Read the model definition and answer for the solid it produces. Units are mm, in the model's axes. Give positions to 0.01 mm unless a question says otherwise; leave off trailing zeros. Write each loop counter-clockwise with the first axis right and the second up, starting at its lowest first coordinate (ties: lowest second). Pieces come first, ordered by that corner, then holes. Notation, with made-up numbers: M -39,62.5 L -29,62.5 A20 cw -29,78.5 Z; hole C 74,51.5 d8. An arc over 180 degrees is marked long. Write each question's results on one line, items separated by ' | '. Start each with the question number.
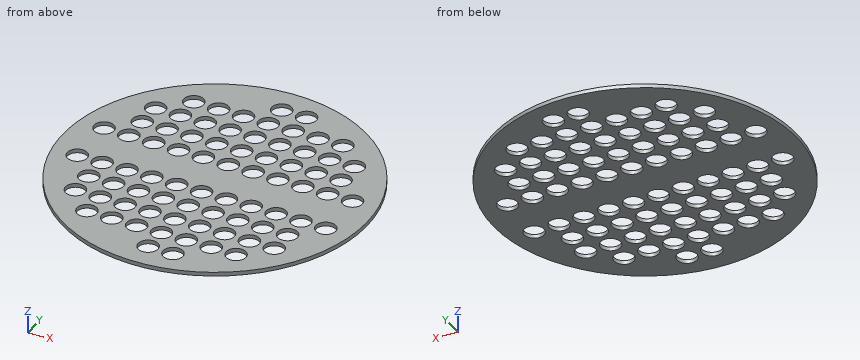
```python
from build123d import *

# Parameters (mm, degrees)
SKETCH1_R           = 193.65
BOSS_EXTRUDE1_DEPTH = 5
SKETCH2_R           = 12.7
CUT_EXTRUDE1_DEPTH  = 274.908095901


with BuildPart() as part:
    # Sketch1 → Boss-Extrude1 (new body)
    with BuildSketch(Plane.XY):
        Circle(SKETCH1_R)
    extrude(amount=BOSS_EXTRUDE1_DEPTH)

    # Sketch2 → Cut-Extrude1 (cut, through all)
    with BuildSketch(Plane.XY.offset(5)):
        with Locations((0, 158.75)):
            Circle(SKETCH2_R)
        with Locations((31.75, 158.75)):
            Circle(SKETCH2_R)
        with Locations((-95.25, 127)):
            Circle(SKETCH2_R)
        with Locations((-63.5, 127)):
            Circle(SKETCH2_R)
        with Locations((-31.75, 127)):
            Circle(SKETCH2_R)
        with Locations((0, 127)):
            Circle(SKETCH2_R)
        with Locations((31.75, 127)):
            Circle(SKETCH2_R)
        with Locations((63.5, 127)):
            Circle(SKETCH2_R)
        with Locations((95.25, 127)):
            Circle(SKETCH2_R)
        with Locations((-63.5, 95.25)):
            Circle(SKETCH2_R)
        with Locations((-31.75, 95.25)):
            Circle(SKETCH2_R)
        with Locations((0, 95.25)):
            Circle(SKETCH2_R)
        with Locations((31.75, 95.25)):
            Circle(SKETCH2_R)
        with Locations((63.5, 95.25)):
            Circle(SKETCH2_R)
        with Locations((95.25, 95.25)):
            Circle(SKETCH2_R)
        with Locations((-63.5, 63.5)):
            Circle(SKETCH2_R)
        with Locations((-31.75, 63.5)):
            Circle(SKETCH2_R)
        with Locations((0, 63.5)):
            Circle(SKETCH2_R)
        with Locations((31.75, 63.5)):
            Circle(SKETCH2_R)
        with Locations((63.5, 63.5)):
            Circle(SKETCH2_R)
        with Locations((95.25, 63.5)):
            Circle(SKETCH2_R)
        with Locations((-63.5, 31.75)):
            Circle(SKETCH2_R)
        with Locations((-31.75, 31.75)):
            Circle(SKETCH2_R)
        with Locations((0, 31.75)):
            Circle(SKETCH2_R)
        with Locations((31.75, 31.75)):
            Circle(SKETCH2_R)
        with Locations((63.5, 31.75)):
            Circle(SKETCH2_R)
        with Locations((95.25, 31.75)):
            Circle(SKETCH2_R)
        with Locations((-95.25, 95.25)):
            Circle(SKETCH2_R)
        with Locations((-95.25, 63.5)):
            Circle(SKETCH2_R)
        with Locations((-95.25, 31.75)):
            Circle(SKETCH2_R)
        with Locations((-127, 95.25)):
            Circle(SKETCH2_R)
        with Locations((-127, 63.5)):
            Circle(SKETCH2_R)
        with Locations((-127, 31.75)):
            Circle(SKETCH2_R)
        with Locations((-158.75, 31.75)):
            Circle(SKETCH2_R)
        with Locations(Location((158.75, 31.75, 0), (0, 0, 180))):
            Circle(SKETCH2_R)
        with Locations(Location((127, 31.75, 0), (0, 0, 180))):
            Circle(SKETCH2_R)
        with Locations(Location((127, 63.5, 0), (0, 0, 180))):
            Circle(SKETCH2_R)
        with Locations(Location((127, 95.25, 0), (0, 0, 180))):
            Circle(SKETCH2_R)
        with Locations((127, -95.25)):
            Circle(SKETCH2_R)
        with Locations((127, -63.5)):
            Circle(SKETCH2_R)
        with Locations((127, -31.75)):
            Circle(SKETCH2_R)
        with Locations((158.75, -31.75)):
            Circle(SKETCH2_R)
        with Locations(Location((-158.75, -31.75, 0), (0, 0, 180))):
            Circle(SKETCH2_R)
        with Locations(Location((-127, -31.75, 0), (0, 0, 180))):
            Circle(SKETCH2_R)
        with Locations(Location((-127, -63.5, 0), (0, 0, 180))):
            Circle(SKETCH2_R)
        with Locations(Location((-127, -95.25, 0), (0, 0, 180))):
            Circle(SKETCH2_R)
        with Locations(Location((-95.25, -31.75, 0), (0, 0, 180))):
            Circle(SKETCH2_R)
        with Locations(Location((-95.25, -63.5, 0), (0, 0, 180))):
            Circle(SKETCH2_R)
        with Locations(Location((-95.25, -95.25, 0), (0, 0, 180))):
            Circle(SKETCH2_R)
        with Locations(Location((95.25, -31.75, 0), (0, 0, 180))):
            Circle(SKETCH2_R)
        with Locations(Location((63.5, -31.75, 0), (0, 0, 180))):
            Circle(SKETCH2_R)
        with Locations(Location((31.75, -31.75, 0), (0, 0, 180))):
            Circle(SKETCH2_R)
        with Locations(Location((0, -31.75, 0), (0, 0, 180))):
            Circle(SKETCH2_R)
        with Locations(Location((-31.75, -31.75, 0), (0, 0, 180))):
            Circle(SKETCH2_R)
        with Locations(Location((-63.5, -31.75, 0), (0, 0, 180))):
            Circle(SKETCH2_R)
        with Locations(Location((95.25, -63.5, 0), (0, 0, 180))):
            Circle(SKETCH2_R)
        with Locations(Location((63.5, -63.5, 0), (0, 0, 180))):
            Circle(SKETCH2_R)
        with Locations(Location((31.75, -63.5, 0), (0, 0, 180))):
            Circle(SKETCH2_R)
        with Locations(Location((0, -63.5, 0), (0, 0, 180))):
            Circle(SKETCH2_R)
        with Locations(Location((-31.75, -63.5, 0), (0, 0, 180))):
            Circle(SKETCH2_R)
        with Locations(Location((-63.5, -63.5, 0), (0, 0, 180))):
            Circle(SKETCH2_R)
        with Locations(Location((95.25, -95.25, 0), (0, 0, 180))):
            Circle(SKETCH2_R)
        with Locations(Location((63.5, -95.25, 0), (0, 0, 180))):
            Circle(SKETCH2_R)
        with Locations(Location((31.75, -95.25, 0), (0, 0, 180))):
            Circle(SKETCH2_R)
        with Locations(Location((0, -95.25, 0), (0, 0, 180))):
            Circle(SKETCH2_R)
        with Locations(Location((-31.75, -95.25, 0), (0, 0, 180))):
            Circle(SKETCH2_R)
        with Locations(Location((-63.5, -95.25, 0), (0, 0, 180))):
            Circle(SKETCH2_R)
        with Locations(Location((95.25, -127, 0), (0, 0, 180))):
            Circle(SKETCH2_R)
        with Locations(Location((63.5, -127, 0), (0, 0, 180))):
            Circle(SKETCH2_R)
        with Locations(Location((31.75, -127, 0), (0, 0, 180))):
            Circle(SKETCH2_R)
        with Locations(Location((0, -127, 0), (0, 0, 180))):
            Circle(SKETCH2_R)
        with Locations(Location((-31.75, -127, 0), (0, 0, 180))):
            Circle(SKETCH2_R)
        with Locations(Location((-63.5, -127, 0), (0, 0, 180))):
            Circle(SKETCH2_R)
        with Locations(Location((-95.25, -127, 0), (0, 0, 180))):
            Circle(SKETCH2_R)
        with Locations(Location((31.75, -158.75, 0), (0, 0, 180))):
            Circle(SKETCH2_R)
        with Locations(Location((0, -158.75, 0), (0, 0, 180))):
            Circle(SKETCH2_R)
    extrude(amount=-CUT_EXTRUDE1_DEPTH, mode=Mode.SUBTRACT)


solid = part.part
```
Item 1: Section A-A, the plane y = -127 is taken. Give the number of separate pieces and of enclosed holes in the cut face, then the cut area to 3 significant figures.
Item 2: Given P1, Ø3, axis at x = 143.5, z = 2, coming from the +Y side; P2, Ø1, axis at x = 114, z = 1, coming from the -Y side; P3, Ø1, axis at y = 37.5, z = 3, coming from the +X side, each flat-ended and moving along its own axis, determine where each tip first touches the part or whether it passes through.
Item 3: Straight lines are drawn through the part: line 1 (X direction, y = 166, z = 0.4); line 2 (Y direction, x = 157, z = 3.2); line 3 (X direction, y = 164, z = 0.5). For each, find the intervals that lie inside material, in ascending order.
Item 4: Section B-B, the plane x = 158.75 is taken. Determine the outline of the cut face in (y, z).
Worked out:
1) separate pieces: 8 | enclosed holes: 0 | area: 573 mm²
2) P1: stops at y = 131.67 | P2: stops at y = -156.9 | P3: stops at x = 190.08
3) line 1: x = -99.72 to -10.43, 10.43 to 21.32, 42.18 to 99.72 | line 2: y = -113.36 to -44.33, -19.17 to 19.17, 44.33 to 113.36 | line 3: x = -102.98 to -11.56, 11.56 to 20.19, 43.31 to 102.98
4) outline: M -110.9,0 L -44.45,0 L -44.45,5 L -110.9,5 Z; M -19.05,0 L 19.05,0 L 19.05,5 L -19.05,5 Z; M 44.45,0 L 110.9,0 L 110.9,5 L 44.45,5 Z
